Geometry: see drawing. Coordinates: mm, zero at the bounding-box minimum. A direction names the side the tool comes from. Round coordinates to 2 decimals unless told otherwise and drop trailing zeros. Order: outer loops, then holes, each group sorted by start corner. A loop starts at its lowest first (then second) coordinate and runs counter-clockwise, first axis right, second up. Notation, with made-up numbers: (-33, -22) -> (6, -22) arc R23 ccw to (6, -11) -> close; hole circle Ø10 at (-17, 15.5). An arc over 180 degrees is marked (long way). Use a Markdown table: item, result.
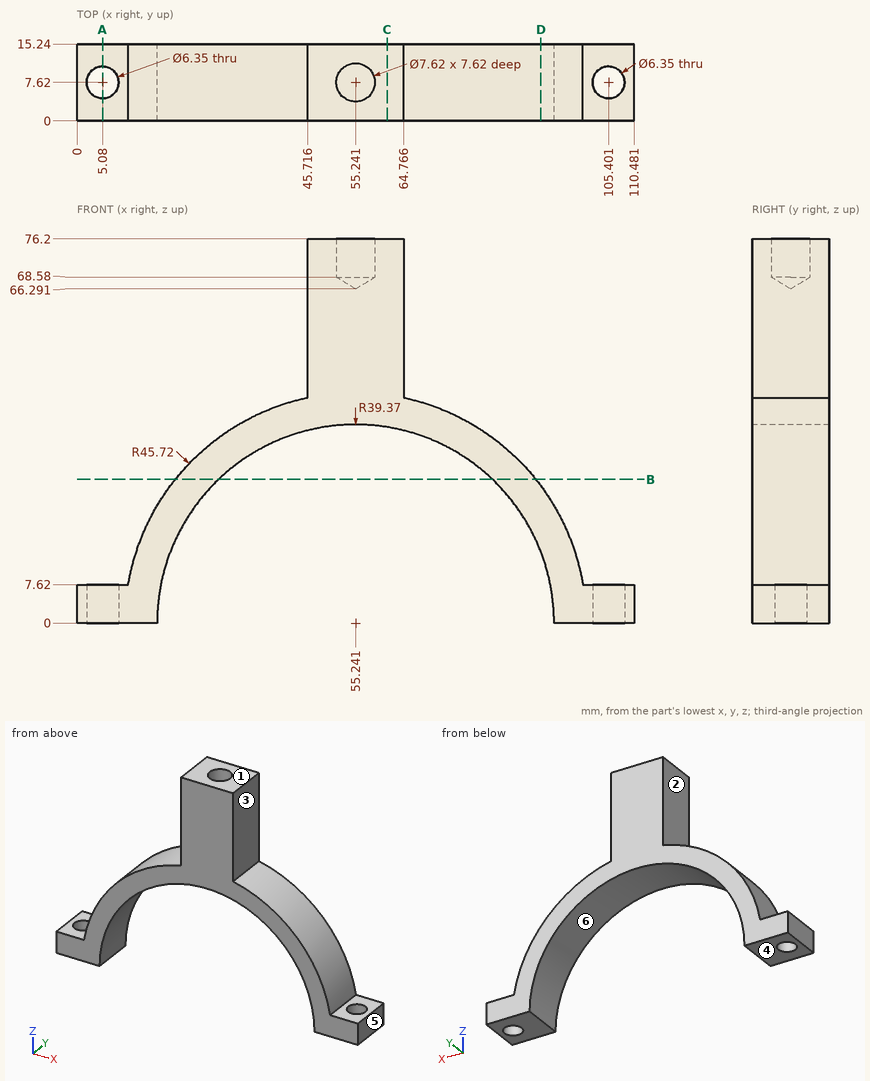
1) Cut plane B-B on z = 28.5. Return loops of the section in (x, y).
Answer key:
| item | result |
|---|---|
| outline | (19.49, 0) -> (28.08, 0) -> (28.08, 15.24) -> (19.49, 15.24) -> close; (82.4, 0) -> (90.99, 0) -> (90.99, 15.24) -> (82.4, 15.24) -> close |
2) Cut plane D-D on x = 92. Return loops of the section in (y, z) (1 decimal).
Answer key:
| item | result |
|---|---|
| outline | (0, 14.1) -> (15.2, 14.1) -> (15.2, 27.2) -> (0, 27.2) -> close |
3) Cut plane A-A on x = 5.08. Return loops of the section in (y, z) (1 decimal).
Answer key:
| item | result |
|---|---|
| outline | (0, 0) -> (4.4, 0) -> (4.4, 7.6) -> (0, 7.6) -> close; (10.8, 0) -> (15.2, 0) -> (15.2, 7.6) -> (10.8, 7.6) -> close |
4) Set-up query: the marked faces 1, 2 and 3. Return all of +Z, -Z, +X, -X, +Y, -Y with unobstructed straight access to the full face (end or side cutting, diameter ignored); none if empty.
Answer key:
| item | result |
|---|---|
| face 1 | +Z, +X, -X, +Y, -Y |
| face 2 | +Z, -X, +Y, -Y |
| face 3 | +Z, +X, +Y, -Y |
5) Ray query, probe 1 along X at (y, z) = (7.62, 2) (1 decimal); probe 2 along X at (y, z) = (7.62, 5.25) (1 decimal); probe 3 along Z at (x, y) = (56, 2.5). Return the intervals inside material, ascending.
Answer key:
| item | result |
|---|---|
| probe 1 | x = 0 to 1.9, 8.3 to 15.9, 94.6 to 102.2, 108.6 to 110.5 |
| probe 2 | x = 0 to 1.9, 8.3 to 16.2, 94.3 to 102.2, 108.6 to 110.5 |
| probe 3 | z = 39.36 to 76.2 |
6) Draft query along X for the marked faces 4, 5 and 6. Return one class per face: released by +X, released by -X, zero draft, split by the parting line, or undercut.
Answer key:
| item | result |
|---|---|
| face 4 | zero draft |
| face 5 | released by +X |
| face 6 | undercut |
7) Contact query for flat-ended pins moving along their axis: P1, Ø8, axis at x = 106, y = 4.5, coming from the +Z side; P2, Ø4, axis at y = 13.5, z = 30, coming from the -X side; P3, Ø7.5, axis at y = 8, z = 65, coming from the +X side. Output: stop coordinate, or through.
Answer key:
| item | result |
|---|---|
| P1 | stops at z = 7.62 |
| P2 | stops at x = 19.1 |
| P3 | stops at x = 64.77 |
8) Cut plane C-C on x = 61.5. Return loops of the section in (y, z), and give its area (3 significant figures).
Answer key:
| item | result |
|---|---|
| outline | (0, 38.87) -> (15.24, 38.87) -> (15.24, 76.2) -> (0, 76.2) -> close |
| area | 569 mm^2 |
